Answer from the drawing. Dimensions are ordinates in mm from the lowest x, y and z of the part. Coordinates: 2 decimals unless noted, no trailing zeros. Write each loop counter-clockwise with the first axis right and the second up, starting at its lowest first coordinate (ties: lowest second). Pieces come first, ordered by that corner, then holes.
(1) The part is cut by section B-B, the plane y = 14.5. Determine the outline of the cut face in (x, z) (1 decimal).
(2) Determine the mould class of the marked faces 1, 2 and 3 for opening direction X: pulls with the +X half, pulls with the -X half, needs draft (parallel to the pull), parting line crosses it, or undercut.
(3) Given pin 1 (12 mm diameter, centred on x = 50, y = 13, fed in from -Z); pin 2 (5 mm diameter, centred on y = 3, z = 44, fed in from -X) (1 decimal); pin 3 (23.5 mm diameter, centred on x = 35.12, z = 35.12, fed in from -Y); pin 4 (10 mm diameter, centred on x = 8.5, z = 37, fed in from -Y), each flat-ended and moving along its own axis, determine where each tip first touches the part or whether it passes through.
(4) Straight lines are drawn through the part: line 1 along X through (y, z) = (9.25, 35); line 2 along Z through (x, y) = (37, 2) (1 decimal); line 3 along X through (y, z) = (3.25, 28) (1 decimal). For each, find the intervals that lie inside material, in ascending order.
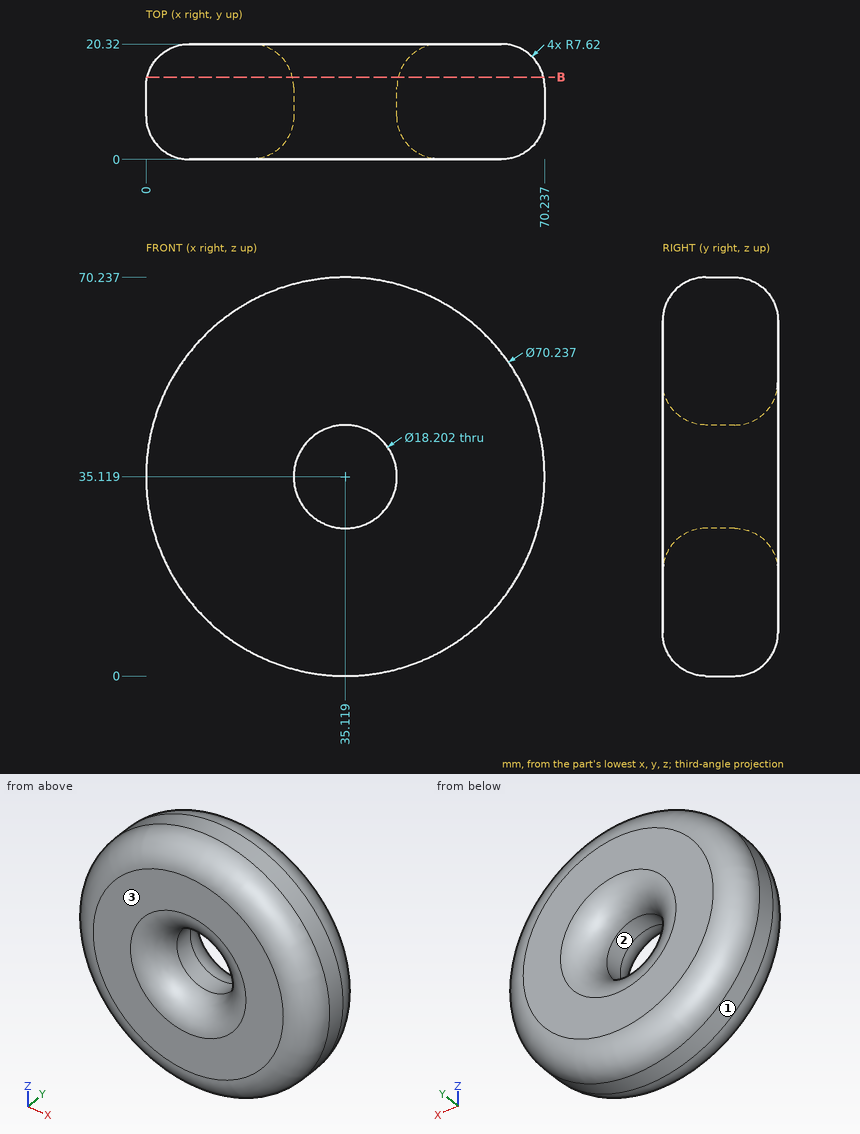
Computed:
1. outline: circle Ø69.8 at (35.1, 35.1); hole circle Ø18.6 at (35.1, 35.1)
2. face 1: parting line crosses it
2. face 2: undercut
2. face 3: needs draft
3. pin 1: stops at z = 1.14
3. pin 2: stops at x = 1.3
3. pin 3: stops at y = 1.84
3. pin 4: stops at y = 0
4. line 1: x = 0 to 26.02, 44.22 to 70.24
4. line 2: z = 2.5 to 23.7, 46.5 to 67.7
4. line 3: x = 2.1 to 27.4, 42.8 to 68.1
